Could you check a few things on this model? Use its own coordinates, in mm. A direction names the side the tool comes from. Give positions to 0.01 mm unless a question says otherwise; leave off trailing zeros. Write each loop counter-clockwise with the first axis right and the second up, starting at its lowest first coordinate (ties: lowest second). Pieces come first, ordered by that corner, then holes. Notation, with made-up numbers: (19, 12) - (72, 12) arc R13 cw to (72, 25) - close; hole circle Ø10 at (84, -36.75). An arc over 180 degrees is marked (long way). Write item = value, one per line.
Solid Edge part; units mm, degrees
sketch "Sketch1" plane through (0, 0, 0) normal (0, -1, 0) x (1, 0, 0)
  circle A0 centre (0, 0) radius 30
extrude "Protrusion1" add sketch "Sketch1" against normal blind 150
sketch "Sketch2" plane through (0, 0, 0) normal (0, -1, 0) x (1, 0, 0)
  circle A0 centre (0, 0) radius 45
extrude "ExtrudedProtrusion_2" add sketch "Sketch2" against normal blind 10
mirror "Mirror1" about plane through (0, 75, 0) normal (0, -1, 0) of "ExtrudedProtrusion_2"
1. I need wall thicknesses on line 1 (Y direction, x = 24, z = 36.5); line 2 (Z direction, x = 1, y = 23); line 3 (X direction, y = 106, z = -9.5). Which ranges of each line are inside material? Lowest first, please.
Filled sheet:
line_1 = 0 to 10, 140 to 150
line_2 = -29.98 to 29.98
line_3 = -28.46 to 28.46
2. Which directions (+Z, -Z, +X, -X, +Y, -Y) give clear straight access to the entire face, cutting with the end or side of a thin tool? Please do faces 4 (the face through (1, 150, -1)), 5 (the face through (-29.97, 74.09, 1.32)).
Filled sheet:
face_4 = +Z, -Z, +X, -X, +Y
face_5 = none
3. If we section it at C-C, the plane z = 0: Please give me the cut outline in (x, y), and give its area (3 significant figures).
Filled sheet:
outline = (-45, 0) - (45, 0) - (45, 10) - (30, 10) - (30, 140) - (45, 140) - (45, 150) - (-45, 150) - (-45, 140) - (-30, 140) - (-30, 10) - (-45, 10) - close
area = 9,600 mm2
4. For pin 1 (5 mm diameter, centred on y = 133, z = 5, fed in from -X); pin 2 (5 mm diameter, centred on x = -32, z = 20.5, fed in from -Y); pin 3 (10 mm diameter, centred on x = -2, y = 54.5, fed in from -Z); pin 4 (3 mm diameter, centred on x = -15.5, y = 17, fed in from +Z), each with a flat end and sliding along its axis, tell me the tip position at first contact or that it passes through.
Filled sheet:
pin_1 = -29.9
pin_2 = 0
pin_3 = -30
pin_4 = 26.53
5. If we section it at B-B, the plane x = 0: Please give me the cut outline in (y, z), and give its area (3 significant figures).
Filled sheet:
outline = (0, -45) - (10, -45) - (10, -30) - (140, -30) - (140, -45) - (150, -45) - (150, 45) - (140, 45) - (140, 30) - (10, 30) - (10, 45) - (0, 45) - close
area = 9,600 mm2
6. If we section it at D-D, the plane y = 90: Please give me the cut outline in (x, z), and give its area (3 significant figures).
Filled sheet:
outline = circle Ø60 at (0, 0)
area = 2,830 mm2
7. If we section it at A-A, the plane z = 39: Please give me the cut outline in (x, y), and give its area (3 significant figures).
Filled sheet:
outline = (-22.45, 0) - (22.45, 0) - (22.45, 10) - (-22.45, 10) - close; (-22.45, 140) - (22.45, 140) - (22.45, 150) - (-22.45, 150) - close
area = 898 mm2
8. Thinking about a two-plate mould opening in Y: for faces 1 (the face through (-9, 10, -29)), 2 (the face through (20.765, 4.93, -39.923)), 3 (the face through (1, 0, 1)), which applies, pulls with the +Y half, pulls with the -Y half, needs draft (parallel to the pull), parting line crosses it, or undercut?
Filled sheet:
face_1 = undercut
face_2 = needs draft
face_3 = pulls with the -Y half
